from build123d import *

# Parameters (mm, degrees)
SKETCH_1_R      = 20
SKETCH_1_R_2    = 1.5
SKETCH_1_R_3    = 3
EXTRUDE_1_DEPTH = 2
SKETCH_3_R      = 11
SKETCH_3_R_2    = 7.5
EXTRUDE_2_DEPTH = 5


with BuildPart() as part:
    # 草图1 → 凸台-拉伸1 (new body)
    with BuildSketch(Plane.XY):
        Circle(SKETCH_1_R)
        with Locations((-12, 12)):
            Circle(SKETCH_1_R_2, mode=Mode.SUBTRACT)
        with Locations((12, 12)):
            Circle(SKETCH_1_R_2, mode=Mode.SUBTRACT)
        with Locations((12, -12)):
            Circle(SKETCH_1_R_2, mode=Mode.SUBTRACT)
        with Locations((-12, -12)):
            Circle(SKETCH_1_R_2, mode=Mode.SUBTRACT)
        Circle(SKETCH_1_R_3, mode=Mode.SUBTRACT)
    extrude(amount=EXTRUDE_1_DEPTH)

    # 草图3 → 凸台-拉伸2 (add)
    with BuildSketch(Plane(origin=(0, 0, 0), x_dir=(-1, 0, 0), z_dir=(0, 0, -1))):
        with Locations(Location((0, 0, 0), (0, 0, 180))):
            Circle(SKETCH_3_R)
        Circle(SKETCH_3_R_2, mode=Mode.SUBTRACT)
    extrude(amount=EXTRUDE_2_DEPTH)


solid = part.part
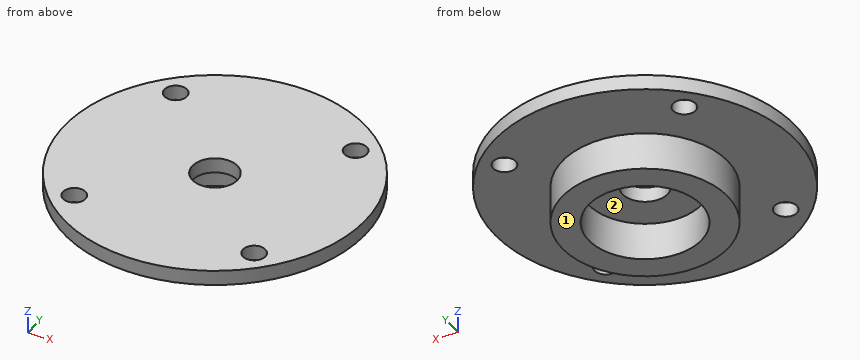
Work out the finished part from the listing and answer in its coordinate system (mm). Face numbers are marked on the shaded views. A direction names the side the tool comes from. Coordinates: 2 decimals unless noted, no trailing zeros. Write each loop counter-clockwise with the first axis right and the second up, starting at its lowest first coordinate (ties: lowest second). Pieces come first, ordered by that corner, then holes. Notation, with made-up numbers: M 34.5,66 L 62.5,66 A13 ccw 62.5,78 Z; hole C 35,9 d7. An arc over 180 degrees is marked long. Use one line per item in the form item = value. Start each with the question number.
1. The part is cut by section C-C (z = 1.25). Give the vertices of the cut face in (x, y).
2. A tool of negligible diameter and unlimited length cuts with its end or side. For the marked faces 1 and 2, from which of +Z, -Z, +X, -X, +Y, -Y can it reach the whole face along a straight path? Write none if from no direction.
3. The part is cut by section A-A (y = 0). Give the vertices of the cut face in (x, z).
4. Each of these flat-tipped pins is pushed along its axis until it touches: P1, Ø3.5, axis at x = -12, y = 12, coming from the +Z side; P2, Ø4, axis at x = 1.5, y = 14, coming from the -Z side; P3, Ø2, axis at x = 0.5, z = -4, coming from the +Y side; P4, Ø4, axis at y = -5.5, z = 1, coming from the -X side. Where does it stop, or does it pass through?
5. The part is cut by section B-B (x = 12). Give the vertices of the cut face in (y, z).
6. Straight lines are drawn through the part: probe 1 along Y at (x, z) = (0, -3.95); probe 2 along X at (y, z) = (11.5, 0.25); probe 3 along Z at (x, y) = (17.5, 1.5). For each, find the intervals that lie inside material, in ascending order. Write a range as from..to.
Evaluation:
q1.outline = C 0,0 d40; hole C -12,-12 d3; hole C -12,12 d3; hole C 0,0 d6; hole C 12,-12 d3; hole C 12,12 d3
q2.face_1 = -Z, +X, -X, +Y, -Y
q2.face_2 = -Z
q3.outline = M -20,0 L -11,0 L -11,-5 L -7.5,-5 L -7.5,0 L -3,0 L -3,2 L -20,2 Z; M 3,0 L 7.5,0 L 7.5,-5 L 11,-5 L 11,0 L 20,0 L 20,2 L 3,2 Z
q4.P1 = 2
q4.P2 = 0
q4.P3 = 11
q4.P4 = -19.69
q5.outline = M -16,0 L -13.5,0 L -13.5,2 L -16,2 Z; M -10.5,0 L 10.5,0 L 10.5,2 L -10.5,2 Z; M 13.5,0 L 16,0 L 16,2 L 13.5,2 Z
q6.probe_1 = -11..-7.5, 7.5..11
q6.probe_2 = -16.36..-13.41, -10.59..10.59, 13.41..16.36
q6.probe_3 = 0..2
